The listing builds one solid part. Answer for the finished solid, in the listing's coordinates (mm). A direction names the side the tool comes from. Round coordinates to 2 decimals unless told otherwise and drop trailing zeros. Write each loop counter-clockwise with the first axis right and the second up, starting at its lowest first coordinate (ties: lowest second). Pieces come first, ordered by that corner, then holes.
(1) A cutting plane is placed at C-C, the plane x = 6. Give the vertices of the cut face in (y, z), and give its area (3 significant figures).
(2) A cutting plane is placed at B-B, the plane z = -7.5. Give the vertices of the cut face in (x, y), and give its area (3 significant figures).
(3) Each of these flat-tipped pins is pushed along its axis until it touches: pin 1 Ø3 at (x, y) = (-25.66, 1.44) entering from -Z; pin 2 Ø1 at (x, z) = (-6.5, -3) entering from -Y; pin 3 Ø13.5 at (x, y) = (-19, 26) entering from -Z. Where does it stop, or does it pass through?
(4) A cutting plane is placed at A-A, the plane y = 33. Give the vertices of the cut face in (x, z), and give its area (3 significant figures).
(5) The mould has two halves that part along Y. Classify faces 1 (the face through (-2.585, 7.041, 1.014)), 2 (the face through (-14.405, 27, 1)), 3 (the face through (-35.085, -2.959, 1.521)), 4 (the face through (-26, 1, 2)): +Y half, -Y half, draft (parallel to the pull), parting line (faces both ways), or undercut.
(6) For faces 5 (the face through (-8, 27, 2)), 6 (the face through (-13, 1.94, -5)), 7 (the face through (-3.155, 26, 1)), determine the directions among +Z, -Z, +X, -X, +Y, -Y from which every point of the face is accessible in a straight line to the end or side of a thin tool.
(7) Find the intervals of material crossed by probe 1 along X at (y, z) = (1.44, -2.75); probe 2 along X at (y, z) = (1.44, 0.4); probe 3 along Z at (x, y) = (-6.5, 38.5), in increasing order.
Autodesk Inventor part; units mm, degrees
ref_plane "YZ Plane" through (0, 0, 0) normal (1, 0, 0) x (0, 1, 0)
ref_plane "XZ Plane" through (0, 0, 0) normal (0, 1, 0) x (-1, 0, 0)
ref_plane "XY Plane" through (0, 0, 0) normal (0, 0, 1) x (1, 0, 0)
sketch "Sketch1" plane through (0, 0, 0) normal (0, 0, 1) x (1, 0, 0)
  line L0 (-35.6553, 6.44) -> (9.3447, 6.44)
  line L1 (9.3447, 6.44) -> (9.3447, -3.56)
  line L2 (9.3447, -3.56) -> (-35.6553, -3.56)
  line L3 (-35.6553, -3.56) -> (-35.6553, 6.44)
  line L4 (-23.1553, 6.44) -> (-3.1553, 6.44)
  line L5 (-3.1553, 6.44) -> (-3.1553, 46.44)
  line L6 (-3.1553, 46.44) -> (-23.1553, 46.44)
  line L7 (-23.1553, 46.44) -> (-23.1553, 6.44)
  point P0 (0, 0)
  dimension "d0" = 20
  dimension "d1" = 10
  dimension "d2" = 40
  dimension "d3" = 12.5
  dimension "d4" = 12.5
  dimension "d5" = 45
extrude "Extrusion1" add sketch "Sketch1" along normal blind 2
sketch "Sketch2" plane through (0, 0, 2) normal (0, 0, 1) x (1, 0, 0)
  circle A0 centre (-25.6553, 1.44) radius 2.6
  circle A1 centre (-0.6553, 1.44) radius 2.6
  line L0 (9.3447, -3.56) -> (9.3447, 6.44)
  line L1 (-35.6553, -3.56) -> (9.3447, -3.56)
  point P0 (0, 0)
  dimension "d8" = 5.2
  dimension "d9" = 10
  dimension "d10" = 25
  dimension "d11" = 5.2
  dimension "d12" = 5
  dimension "d13" = 5
extrude "Extrusion2" cut sketch "Sketch2" against normal blind 2
sketch "Sketch3" plane through (0, 0, 2) normal (0, 0, 1) x (1, 0, 0)
  line L0 (-35.6553, -3.56) -> (9.3447, -3.56)
  line L1 (9.3447, -3.56) -> (9.3447, 6.44)
  line L2 (9.3447, 6.44) -> (-35.6553, 6.44)
  line L3 (-35.6553, 6.44) -> (-35.6553, -3.56)
  point P0 (0, 0)
extrude "Extrusion3" add sketch "Sketch3" along normal blind 1
sketch "Sketch4" plane through (0, 0, 2) normal (0, 0, 1) x (1, 0, 0)
  line L0 (-23.1553, 6.44) -> (-3.1553, 6.44)
  line L1 (-14.4053, 6.44) -> (-11.9053, 6.44)
  line L2 (-11.9053, 6.44) -> (-11.9053, 46.44)
  line L3 (-11.9053, 46.44) -> (-14.4053, 46.44)
  line L4 (-14.4053, 46.44) -> (-14.4053, 6.44)
  line L5 (-23.1553, 46.44) -> (-23.1553, 6.44)
  line L6 (-3.1553, 6.44) -> (-3.1553, 46.44)
  point P0 (0, 0)
  dimension "d18" = 2.5
  dimension "d19" = 40
  dimension "d20" = 8.75
  dimension "d21" = 8.75
extrude "Extrusion4" cut sketch "Sketch4" against normal blind 2
fillet "Fillet1" radius 2 6 edges at (-35.6553, 6.44, 1.5) (9.3447, 6.44, 1.5) (-3.1553, 46.44, 1) (-23.1553, 46.44, 1) (-3.1553, 6.44, 1) (-23.1553, 6.44, 1)
fillet "Fillet2" radius 2 2 edges at (9.3447, -3.56, 1.5) (-35.6553, -3.56, 1.5)
sketch "Sketch5" plane through (0, 0, 0) normal (0, 0, -1) x (-1, 0, 0)
  circle A0 centre (0.6553, 1.44) radius 2.6
  circle A1 centre (0.6553, 1.44) radius 2.6
  circle A2 centre (25.6553, 1.44) radius 2.6
  circle A3 centre (25.6553, 1.44) radius 2.6
  circle A4 centre (25.6553, 1.44) radius 3.6
  circle A5 centre (0.6553, 1.44) radius 3.6
  point P0 (0, 0)
  dimension "d26" = 7.2
  dimension "d27" = 7.2
extrude "Extrusion5" add sketch "Sketch5" along normal blind 10
sketch "Sketch6" plane through (0, 0, 0) normal (0, 0, -1) x (-1, 0, 0)
  line L0 (3.6821, 0.94) -> (22.6767, 0.94)
  line L1 (22.6767, 0.94) -> (22.6767, 1.94)
  line L2 (22.6767, 1.94) -> (3.6821, 1.94)
  line L3 (3.6821, 1.94) -> (3.6821, 0.94)
  circle A0 centre (0.6553, 1.44) radius 2.6
  point P0 (0, 0)
  dimension "d30" = 0.5
  dimension "d31" = 0.5
extrude "Extrusion6" add sketch "Sketch6" along normal blind 10 contours L3 L2 L1 L0
properties part number "Top Tube Holder"
Solutions:
1. outline: (-3.56, 0) - (6.44, 0) - (6.44, 3) - (-3.56, 3) - close
1. area: 30.0 mm2
2. outline: (-22.09, 0.94) - (-4.22, 0.94) arc R3.6 ccw (long way) to (-4.22, 1.94) - (-22.09, 1.94) arc R3.6 ccw (long way) to start; hole circle Ø5.2 at (-25.66, 1.44); hole circle Ø5.2 at (-0.66, 1.44)
2. area: 56.8 mm2
3. pin 1: stops at z = 2
3. pin 2: stops at y = 0.94
3. pin 3: stops at z = 0
4. outline: (-23.16, 0) - (-14.41, 0) - (-14.41, 2) - (-23.16, 2) - close; (-11.91, 0) - (-3.16, 0) - (-3.16, 2) - (-11.91, 2) - close
4. area: 35.0 mm2
5. face 1: +Y half
5. face 2: draft
5. face 3: -Y half
5. face 4: undercut
6. face 5: +Z, +X, -X, +Y
6. face 6: -Z, +Y
6. face 7: +Z, -Z, +X, +Y
7. probe 1: x = -29.26 to -28.26, -23.06 to -3.26, 1.94 to 2.94
7. probe 2: x = -35.66 to -28.26, -23.06 to -3.26, 1.94 to 9.34
7. probe 3: z = 0 to 2
